CAD build for the part. Positions are in the model's coordinates, mm. Face numbers are marked on the shaded views. A direction names the side the tool comes from. Coordinates: 2 decimals unless noted, no trailing zeros. Write each loop counter-clockwise with the first axis right and the second up, starting at its lowest first coordinate (ties: lowest second). Pieces come first, ordered by that corner, then holes. Notation, with made-up numbers: (-10, 42.25) - (39, 42.25) arc R20 cw to (39, 46.25) - close; hole circle Ø11 at (51.25, 30). An arc over 180 degrees is marked (long way). Answer in a Markdown table with one row per item. Add a question column.
Q1. Band-saw the part on A-A (x = -50). List the corners of the cut face in (y, z), and give its area (3 significant figures).
Q2. Two-plate mould, pull along Z, no slides. Class the marked faces 1, 2, 3 and 4: +Z half, -Z half, draft (parallel to the pull), parting line (faces both ways), or undercut.
Q3. Pin check, flat tips, straight feed: pin 1 (4 mm diameter, centred on x = -28.5, z = 7, fed in from -Y); pin 2 (1 mm diameter, centred on x = -1, z = 21.5, fed in from -Y); pin 3 (6 mm diameter, centred on x = -17, z = 23, fed in from +Y); pin 4 (10 mm diameter, centred on x = 13, y = 8, fed in from +Z). Stop position of each tip, or through.
Q4. Drill centre lines: line 1 along X through (y, z) = (4, 26.5); line 2 along X through (y, z) = (13, 41); line 3 along X through (y, z) = (2, 38). Where is each one in solid material? Low to high. Write a range as from..to.
Q5. Band-saw the part on D-D (x = -19). List the corners of the cut face in (y, z).
Q6. Band-saw the part on B-B (y = 4). List the corners of the cut face in (x, z), and give its area (3 significant figures).
Q7. 3-axis set-ups, long thin cutter, end or side, ignore diameter. For the marked faces 5, 6, 7 and 8: which of +Z, -Z, +X, -X, +Y, -Y reach the whole face in a straight line?
```python
from build123d import *

# Parameters (mm, degrees)
F0_W          = 58.5
F0_H          = 1.5
F0_H_2        = 3
F1_DEPTH      = 50
F9_DEPTH      = 10
F10_T1_DEPTH  = 28
F10_T3_DEPTH  = 14
F10_T5_DEPTH  = 14
F10_T10_DEPTH = 28
F10_T16_DEPTH = 28
F11_R         = 0.5
F11_R_2       = 1
F11_R_3       = 1.5
F11_R_4       = 2
F11_R_5       = 2.5
F11_R_6       = 3
F11_R_7       = 3.5
F12_DEPTH     = 3
F13_W         = 5
F13_H         = 2
F14_W         = 5
F14_H         = 4
F15_DEPTH     = 1
F16_DEPTH     = 2
F17_DEPTH     = 3
F18_DEPTH     = 4
F19_DEPTH     = 5


# Not quite as in the source:
# - a fillet or chamfer that OpenCascade refuses, or shapes differently, is made with other operations: its cross-section is extruded or revolved along the edge and cut away or added


with BuildPart() as f1:
    # F0 (on Top) → F1 (new body)
    with BuildSketch(Plane.XY):
        with Locations((-30.75, -0.75)):
            Rectangle(F0_W, F0_H)
        with Locations((-30.75, 0.75)):
            Rectangle(F0_W, F0_H)
        Polygon((1.5, 1.5), (-1.5, 1.5), (-1.5, 0), (-1.5, -1.5), (1.5, -1.5), align=None)
        with Locations((30.75, 0)):
            Rectangle(F0_W, F0_H_2)
    extrude(amount=F1_DEPTH)

    # F4 (on offset) + F5 (on offset) + F6 (on Right) + F7 (on face) + F8 (on face) → F9 (join, symmetric)
    with BuildSketch(Plane.YZ.offset(50)):
        Polygon((0, 23.3904352013), (0, 0), (16.9536601964, 46.5797985667), (7.5567339886, 50), (0, 29.2380440016), align=None)
        Polygon((-9.4361192301, 49.3159597133), (0, 23.3904352013), (0, 29.2380440016), (-7.5567339886, 50), align=None)
    with BuildSketch(Plane.YZ.offset(25)):
        Polygon((0, 29.0621284988), (0, 10.1325158336), (16.6198118589, 45.7738173826), (7.5567339886, 50), (0, 33.7945316651), align=None)
        Polygon((-9.3693495626, 49.1547634765), (0, 29.0621284988), (0, 33.7945316651), (-7.5567339886, 50), align=None)
    with BuildSketch(Plane.YZ):
        Polygon((0, 32.9113527925), (0, 16.9113527925), (16.2169880264, 45), (7.5567339886, 50), (0, 36.9113527925), align=None)
        Polygon((-9.2887847961, 49), (0, 32.9113527925), (0, 36.9113527925), (-7.5567339886, 50), align=None)
    with BuildSketch(Plane(origin=(-25, 0, 0), x_dir=(0, -1, 0), z_dir=(-1, 0, 0))):
        Polygon((-15.7482544314, 44.2642356365), (0, 21.7733974606), (0, 35.7209718255), (0, 39.2078654168), (-7.5567339886, 50), align=None)
        Polygon((0, 39.2078654168), (0, 35.7209718255), (9.1950380771, 48.8528471273), (7.5567339886, 50), align=None)
    with BuildSketch(Plane(origin=(-50, 0, 0), x_dir=(0, -1, 0), z_dir=(-1, 0, 0))):
        Polygon((-15.2171784197, 43.5721239031), (0, 25.4369968523), (0, 37.8827874671), (0, 40.9942351209), (-7.5567339886, 50), align=None)
        Polygon((0, 40.9942351209), (0, 37.8827874671), (9.0888228748, 48.7144247806), (7.5567339886, 50), align=None)
    extrude(amount=F9_DEPTH, both=True, dir=(1, 0, 0))

    # F10: fillet of radius 5 on 5 edges, made by hand

    # F10_s2 → F10_t1 (cut)
    with BuildSketch(Plane.XZ.offset(-14)):
        with BuildLine():
            ThreePointArc((-55, 0), (-58.5355339059, 1.4644660941), (-60, 5))
            Line((-60, 5), (-60, 0))
            Line((-60, 0), (-55, 0))
        make_face()
    extrude(amount=F10_T1_DEPTH, mode=Mode.SUBTRACT)

    # F10_s4 → F10_t3 (cut)
    with BuildSketch(Plane.XZ):
        with BuildLine():
            ThreePointArc((55, 0), (58.5355339059, 1.4644660941), (60, 5))
            Line((60, 5), (60, 0))
            Line((60, 0), (55, 0))
        make_face()
    extrude(amount=F10_T3_DEPTH, mode=Mode.SUBTRACT)

    # F10_s6 → F10_t5 (cut)
    with BuildSketch(Plane.XZ.offset(-14)):
        with BuildLine():
            ThreePointArc((55, 0), (58.5355339059, 1.4644660941), (60, 5))
            Line((60, 5), (60, 0))
            Line((60, 0), (55, 0))
        make_face()
    extrude(amount=F10_T5_DEPTH, mode=Mode.SUBTRACT)


with BuildPart() as f10_tool8:
    # F10_s9 → F10_t10 (new body)
    with BuildSketch(Plane.XZ.offset(14)):
        with BuildLine():
            ThreePointArc((60, 45), (58.5355339059, 48.5355339059), (55, 50))
            Line((55, 50), (60, 50))
            Line((60, 50), (60, 45))
        make_face()
    extrude(amount=-F10_T10_DEPTH)

    split(bisect_by=Plane(origin=(0, 9.3969262079, 3.4202014333), x_dir=(1, 0, 0), z_dir=(0, 0.9396926208, 0.3420201433)), keep=Keep.TOP)

    split(bisect_by=Plane(origin=(0, -9.3969262079, 3.4202014333), x_dir=(1, 0, 0), z_dir=(0, -0.9396926208, 0.3420201433)), keep=Keep.TOP)


with BuildPart() as f1_1:
    add(f1.part)

    # F10_t7: cut F10_tool8
    add(f10_tool8.part, mode=Mode.SUBTRACT)


with BuildPart() as f10_tool14:
    # F10_s15 → F10_t16 (new body)
    with BuildSketch(Plane.XZ.offset(-14)):
        with BuildLine():
            ThreePointArc((-55, 50), (-58.5355339059, 48.5355339059), (-60, 45))
            Line((-60, 45), (-60, 50))
            Line((-60, 50), (-55, 50))
        make_face()
    extrude(amount=F10_T16_DEPTH)

    split(bisect_by=Plane(origin=(0, 20.1857202879, 16.9378304486), x_dir=(1, 0, 0), z_dir=(0, 0.7660444431, 0.6427876097)), keep=Keep.TOP)

    split(bisect_by=Plane(origin=(0, -20.1857202879, 16.9378304486), x_dir=(1, 0, 0), z_dir=(0, -0.7660444431, 0.6427876097)), keep=Keep.TOP)


with BuildPart() as f1_2:
    add(f1_1.part)

    # F10_t13: cut F10_tool14
    add(f10_tool14.part, mode=Mode.SUBTRACT)

    # F11 (on face) → F12 (cut, through all)
    with BuildSketch(Plane(origin=(0, 1.5, 0), x_dir=(-1, 0, 0), z_dir=(0, 1, 0))):
        with Locations((25, 5.4156194707)):
            Circle(F11_R)
        with Locations((25, 8.9156194707)):
            Circle(F11_R_2)
        with Locations((25, 13.4156194707)):
            Circle(F11_R_3)
        with Locations((25, 18.9156194707)):
            Circle(F11_R_4)
        with Locations((50, 4.7246272412)):
            Circle(F11_R_5)
        with Locations((50, 12.2246272412)):
            Circle(F11_R_6)
        with Locations((50, 20.7246272412)):
            Circle(F11_R_7)
    extrude(amount=-F12_DEPTH, mode=Mode.SUBTRACT)

    # F13 (on face) + F14 (on face) → F15 (join)
    with BuildSketch(Plane.XZ.offset(1.5)):
        with Locations((0, 6.5094290039)):
            Rectangle(F13_W, F13_H)
    with BuildSketch(Plane.XZ.offset(1.5)):
        with Locations((25, 5.2788888796)):
            Rectangle(F14_W, F14_H)
    extrude(amount=F15_DEPTH)

    # F13 (on face) + F14 (on face) → F16 (join)
    with BuildSketch(Plane.XZ.offset(1.5)):
        with Locations((0, 11.5094290039)):
            Rectangle(F13_W, F13_H)
    with BuildSketch(Plane.XZ.offset(1.5)):
        with Locations((25, 12.2788888796)):
            Rectangle(F14_W, F14_H)
    extrude(amount=F16_DEPTH)

    # F13 (on face) + F14 (on face) → F17 (join)
    with BuildSketch(Plane.XZ.offset(1.5)):
        with Locations((0, 16.5094290039)):
            Rectangle(F13_W, F13_H)
    with BuildSketch(Plane.XZ.offset(1.5)):
        with Locations((25, 19.2788888796)):
            Rectangle(F14_W, F14_H)
    extrude(amount=F17_DEPTH)

    # F13 (on face) + F14 (on face) → F18 (join)
    with BuildSketch(Plane.XZ.offset(1.5)):
        with Locations((0, 21.5094290039)):
            Rectangle(F13_W, F13_H)
    with BuildSketch(Plane.XZ.offset(1.5)):
        with Locations((25, 26.2788888796)):
            Rectangle(F14_W, F14_H)
    extrude(amount=F18_DEPTH)

    # F13 (on face) → F19 (join)
    with BuildSketch(Plane.XZ.offset(1.5)):
        with Locations((0, 26.5094290039)):
            Rectangle(F13_W, F13_H)
    extrude(amount=F19_DEPTH)


solid = f1_2.part
```
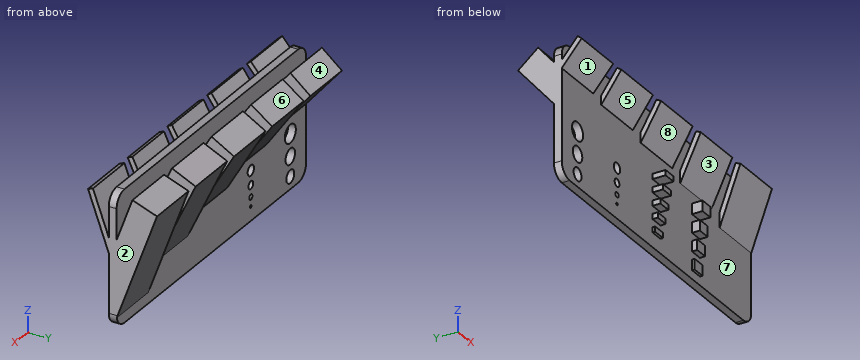
Checked values:
| question | item | result |
|---|---|---|
| 1 | outline | (-9.09, 48.71) - (-1.5, 39.67) - (-1.5, 24.22) - (1.5, 24.22) - (1.5, 27.22) - (15.22, 43.57) - (7.56, 50) - (1.5, 42.78) - (1.5, 50) - (-1.5, 50) - (-1.5, 42.78) - (-7.56, 50) - close; (-1.5, 0) - (1.5, 0) - (1.5, 2.22) - (-1.5, 2.22) - close; (-1.5, 7.22) - (1.5, 7.22) - (1.5, 9.22) - (-1.5, 9.22) - close; (-1.5, 15.22) - (1.5, 15.22) - (1.5, 17.22) - (-1.5, 17.22) - close |
| 1 | area | 271 mm² |
| 2 | face 1 | -Z half |
| 2 | face 2 | draft |
| 2 | face 3 | undercut |
| 2 | face 4 | +Z half |
| 3 | pin 1 | stops at y = -1.5 |
| 3 | pin 2 | stops at y = -5.5 |
| 3 | pin 3 | stops at y = 2.96 |
| 3 | pin 4 | stops at z = 50 |
| 4 | line 1 | x = -10..10, 15..35, 40..60 |
| 4 | line 2 | x = -60..-40, -35..-15, -10..10, 15..35, 40..60 |
| 4 | line 3 | x = -60..-40, -35..-15, -10..10, 15..35 |
| 5 | outline | (-9.2, 48.85) - (-1.5, 37.86) - (-1.5, 0) - (1.5, 0) - (1.5, 23.92) - (15.75, 44.26) - (7.56, 50) - (1.5, 41.35) - (1.5, 50) - (-1.5, 50) - (-1.5, 41.35) - (-7.56, 50) - close |
| 6 | outline | (-60, 30.2) - (-40, 30.2) - (-40, 45.76) - (-60, 45.76) - close; (-35, 27.49) - (-15, 27.49) - (-15, 44.92) - (-35, 44.92) - close; (-10, 23.84) - (10, 23.84) - (10, 43.84) - (-10, 43.84) - close; (15, 18.71) - (35, 18.71) - (35, 42.37) - (15, 42.37) - close; (40, 10.99) - (60, 10.99) - (60, 40.23) - (40, 40.23) - close |
| 6 | area | 2,120 mm² |
| 7 | face 5 | -Z, -X, -Y |
| 7 | face 6 | +Z, -X, +Y |
| 7 | face 7 | none |
| 7 | face 8 | -X, -Y |
